Design review of the part built by this model. Coordinates are the model's own, in mm. Coordinates: 2 decimals unless noted, no trailing zeros. Order: outer loops, then holes, each group sorted by start corner. A loop starts at its lowest first (then second) coordinate and runs counter-clockwise, first axis right, second up.
from build123d import *

# Parameters (mm, degrees)
ESQUISSE2_R        = 6.4135
BOSS_EXTRU_1_DEPTH = 6.35


with BuildPart() as part:
    # Esquisse2 → Boss.-Extru.1 (new body)
    with BuildSketch(Plane(origin=(-37.908707754, 0, 1.245941937), x_dir=(1, 0, 0), z_dir=(0, 0, 1))):
        with BuildLine():
            Line((39.610752218, -12.665274164), (61.291934706, -59.160720054))
            ThreePointArc((61.291934706, -59.160720054), (61.826338046, -59.99956527), (62.559641152, -60.671513766))
            Line((62.559641152, -60.671513766), (72.053336788, -67.319071016))
            ThreePointArc((72.053336788, -67.319071016), (74.008942258, -69.522860983), (74.759386744, -72.372056668))
            ThreePointArc((74.759386744, -72.372056668), (94.394175617, -78.311143591), (82.097766158, -61.891764736))
            ThreePointArc((82.097766158, -61.891764736), (79.163730867, -62.161059907), (76.423989233, -61.077132438))
            Line((76.423989233, -61.077132438), (69.160323465, -55.991058912))
            ThreePointArc((69.160323465, -55.991058912), (67.938151622, -54.871144752), (67.047479388, -53.473069393))
            Line((67.047479388, -53.473069393), (46.516817555, -9.444923009))
            ThreePointArc((46.516817555, -9.444923009), (45.921882482, -6.749760897), (46.526606303, -4.056778228))
            ThreePointArc((46.526606303, -4.056778228), (33.883268811, 8.632581672), (35.476901763, -9.209340075))
            ThreePointArc((35.476901763, -9.209340075), (37.928555152, -10.477110645), (39.610752218, -12.665274164))
        make_face()
        with Locations((37.908707754, 0)):
            Circle(ESQUISSE2_R, mode=Mode.SUBTRACT)
        with Locations((85.551429299, -72.11938596)):
            Circle(ESQUISSE2_R, mode=Mode.SUBTRACT)
    extrude(amount=BOSS_EXTRU_1_DEPTH)


solid = part.part
1. Add section A-A (y = 0). Give the boundary of the cut face in (x, z) (1 decimal).
2. Insertion check: pin 1 (1 mm diameter, centred on x = 23, z = 4, fed in from -Y); pin 2 (2 mm diameter, centred on x = 20.5, z = 2.5, fed in from +Y). Each pin has a flat end and moves straight along its axis. Give the tip position at first contact, or say it passes through.
3. Add section B-B (x = 0). Give the boundary of the cut face in (y, z) (1 decimal).
4. To check wall thickness, follow line 1 (Y direction, x = 0, z = 4.5) (1 decimal); line 2 (X direction, y = -76, z = 7); line 3 (Y direction, x = 49, z = 7.25). State the ranges of each line that lie inside material, in increasing order.
5. Add section C-C (z = 2.75). State how many separate pieces and enclosed holes the cut face has, and give its area (3 significant figures).
6. Add section D-D (x = 19). Give the boundary of the cut face in (y, z).
7. Mouldability with a two-part tool opening along X and no side actions: class faces 1 (the flat face through (34.934, -58.57, 4.376)), 2 (the cylindrical face through (-3.727, 8.765, 4.376)), 3 (the cylindrical face through (6.117, 1.926, 4.376)), 4 (the cylindrical face through (41.296, -62.167, 4.376)) as pulls with the +X half, pulls with the -X half, needs draft (parallel to the pull), parting line crosses it, or undercut.
Solution:
1. outline: (-9.5, 1.2) - (-6.4, 1.2) - (-6.4, 7.6) - (-9.5, 7.6) - close; (6.4, 1.2) - (9.5, 1.2) - (9.5, 7.6) - (6.4, 7.6) - close
2. pin 1: stops at y = -59.39
2. pin 2: stops at y = -32.8
3. outline: (-10.5, 1.2) - (-6.4, 1.2) - (-6.4, 7.6) - (-10.5, 7.6) - close; (6.4, 1.2) - (9.5, 1.2) - (9.5, 7.6) - (6.4, 7.6) - close
4. line 1: y = -10.5 to -6.4, 6.4 to 9.5
4. line 2: x = 37.57 to 42.54, 52.75 to 57.72
4. line 3: y = -82.83 to -78.39, -65.85 to -61.41
5. separate pieces: 1
5. enclosed holes: 2
5. area: 926 mm2
6. outline: (-49.76, 1.25) - (-31.73, 1.25) - (-31.73, 7.6) - (-49.76, 7.6) - close
7. face 1: pulls with the +X half
7. face 2: parting line crosses it
7. face 3: undercut
7. face 4: undercut
